The model under review builds one solid part; all positions refer to its coordinate system, in mm. Face numbers are marked on the shaded views. A direction names the side the tool comes from. Round coordinates to 2 decimals unless told otherwise and drop trailing zeros. Loops run counter-clockwise (first coordinate to the right, second up) from the corner with the lowest first, then second, coordinate; pieces in that order, holes last. Notation, with made-up numbers: (5.25, 7.25) -> (25.25, 7.25) arc R20 cw to (25.25, 14.25) -> close; hole circle Ø1 at (42.5, 29). An arc over 180 degrees is marked (long way). Use a Markdown table: item, result. Add a question column.
1) Consider section C-C on x = 4. Give the boundary of the cut face in (y, z).
2) Mouldability with a two-part tool opening along X and no side actions: class the marked faces 1, 2 and 3 as released by +X, released by -X, zero draft, split by the parting line, or undercut.
3) Consider section B-B on y = -1.5. Give the boundary of the cut face in (x, z).
4) Consider section D-D on x = -9.5. Give the boundary of the cut face in (y, z), plus the area to 3 significant figures.
5) Wall thickness on probe 1 along Y at (x, z) = (-24.5, -3.5); probe 2 along X at (y, z) = (-1, -15): over which ranges is each line inside the solid? List them lowest first.
6) For the marked faces 4, 5 and 6, list the 3-axis set-ups (+Z, -Z, +X, -X, +Y, -Y) from which the entire face can be reached by the end or side of a thin tool; tool diameter is ignored.
7) Consider section A-A on z = 13.5. Give the boundary of the cut face in (x, y), plus the area to 3 significant figures.
from build123d import *

# Parameters (mm, degrees)
SKETCH1_W           = 74.8284
SKETCH1_H           = 43.18
BOSS_EXTRUDE1_DEPTH = 21.59
SKETCH12_W          = 15.494
SKETCH12_H          = 15.494
CUT_EXTRUDE1_DEPTH  = 62.077515189
SKETCH15_W          = 15.494
SKETCH15_H          = 15.494
CUT_EXTRUDE2_DEPTH  = 62.077515189
SKETCH16_W          = 15.494
SKETCH16_H          = 15.494
CUT_EXTRUDE3_DEPTH  = 81.817978486


with BuildPart() as part:
    # Sketch1 → Boss-Extrude1 (new, symmetric)
    with BuildSketch(Plane(origin=(0, 0, 0), x_dir=(1, 0, 0), z_dir=(0, 1, 0))):
        Rectangle(SKETCH1_W, SKETCH1_H)
    extrude(amount=BOSS_EXTRUDE1_DEPTH, both=True)

    # Sketch12 → Cut-Extrude1 (cut, through all)
    with BuildSketch(Plane(origin=(0, 21.59, 0), x_dir=(1, 0, 0), z_dir=(0, 1, 0))):
        Rectangle(SKETCH12_W, SKETCH12_H)
    extrude(amount=-CUT_EXTRUDE1_DEPTH, mode=Mode.SUBTRACT)

    # Sketch15 → Cut-Extrude2 (cut, through all)
    with BuildSketch(Plane.XY.offset(21.59)):
        Rectangle(SKETCH15_W, SKETCH15_H)
    extrude(amount=-CUT_EXTRUDE2_DEPTH, mode=Mode.SUBTRACT)

    # Sketch16 → Cut-Extrude3 (cut, through all)
    with BuildSketch(Plane(origin=(37.4142, 0, 0), x_dir=(0, 0, -1), z_dir=(1, 0, 0))):
        Rectangle(SKETCH16_W, SKETCH16_H)
    extrude(amount=-CUT_EXTRUDE3_DEPTH, mode=Mode.SUBTRACT)


solid = part.part
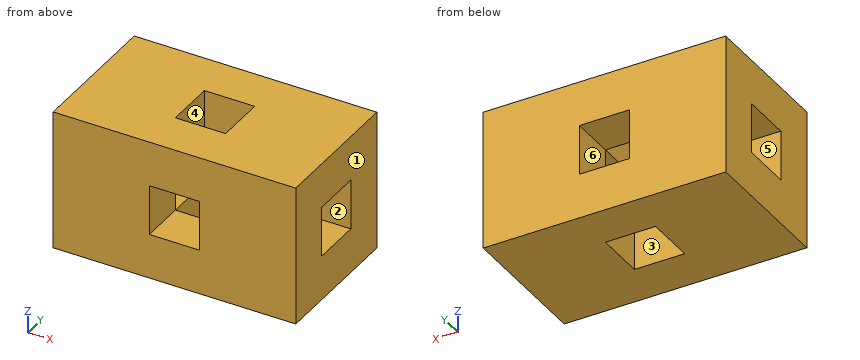
Result set:
| question | item | result |
|---|---|---|
| 1 | outline | (-21.59, -21.59) -> (-7.75, -21.59) -> (-7.75, -7.75) -> (-21.59, -7.75) -> close; (-21.59, 7.75) -> (-7.75, 7.75) -> (-7.75, 21.59) -> (-21.59, 21.59) -> close; (7.75, -21.59) -> (21.59, -21.59) -> (21.59, -7.75) -> (7.75, -7.75) -> close; (7.75, 7.75) -> (21.59, 7.75) -> (21.59, 21.59) -> (7.75, 21.59) -> close |
| 2 | face 1 | released by +X |
| 2 | face 2 | zero draft |
| 2 | face 3 | undercut |
| 3 | outline | (-37.41, -21.59) -> (-7.75, -21.59) -> (-7.75, -7.75) -> (-37.41, -7.75) -> close; (-37.41, 7.75) -> (-7.75, 7.75) -> (-7.75, 21.59) -> (-37.41, 21.59) -> close; (7.75, -21.59) -> (37.41, -21.59) -> (37.41, -7.75) -> (7.75, -7.75) -> close; (7.75, 7.75) -> (37.41, 7.75) -> (37.41, 21.59) -> (7.75, 21.59) -> close |
| 4 | outline | (-21.59, -21.59) -> (21.59, -21.59) -> (21.59, 21.59) -> (-21.59, 21.59) -> close; hole (-7.75, -7.75) -> (7.75, -7.75) -> (7.75, 7.75) -> (-7.75, 7.75) -> close |
| 4 | area | 1,620 mm2 |
| 5 | probe 1 | -21.59 to -7.75, 7.75 to 21.59 |
| 5 | probe 2 | -37.41 to -7.75, 7.75 to 37.41 |
| 6 | face 4 | +Z, -Z |
| 6 | face 5 | +X, -X |
| 6 | face 6 | +Y, -Y |
| 7 | outline | (-37.41, -21.59) -> (37.41, -21.59) -> (37.41, 21.59) -> (-37.41, 21.59) -> close; hole (-7.75, -7.75) -> (7.75, -7.75) -> (7.75, 7.75) -> (-7.75, 7.75) -> close |
| 7 | area | 2,990 mm2 |
